from build123d import *

# Parameters (mm, degrees)
F0_W     = 8
F0_H     = 24
F1_DEPTH = 4
F2_DEPTH = 8
F3_W     = 16
F3_H     = 16
F4_DEPTH = 2


with BuildPart() as f1:
    # F0 (on Front) → F1 (new body, symmetric)
    with BuildSketch(Plane.XZ):
        with Locations((-4, 7)):
            Rectangle(F0_W, F0_H)
        with Locations((-12, 7)):
            Rectangle(F0_W, F0_H)
        with Locations((4, 7)):
            Rectangle(F0_W, F0_H)
        with Locations((12, 7)):
            Rectangle(F0_W, F0_H)
        with Locations((4, -17)):
            Rectangle(F0_W, F0_H)
        with Locations((-4, -17)):
            Rectangle(F0_W, F0_H)
    extrude(amount=F1_DEPTH, both=True)

    # F0 (on Front) → F2 (join, symmetric)
    with BuildSketch(Plane.XZ):
        Polygon((-8, 19), (0, 19), (8, 19), (8, 35), (-8, 35), align=None)
    extrude(amount=F2_DEPTH, both=True)

    # F3 (on face) → F4 (join)
    with BuildSketch(Plane(origin=(0, 0, -29), x_dir=(1, 0, 0), z_dir=(0, 0, -1))):
        Rectangle(F3_W, F3_H)
    extrude(amount=F4_DEPTH)


solid = f1.part
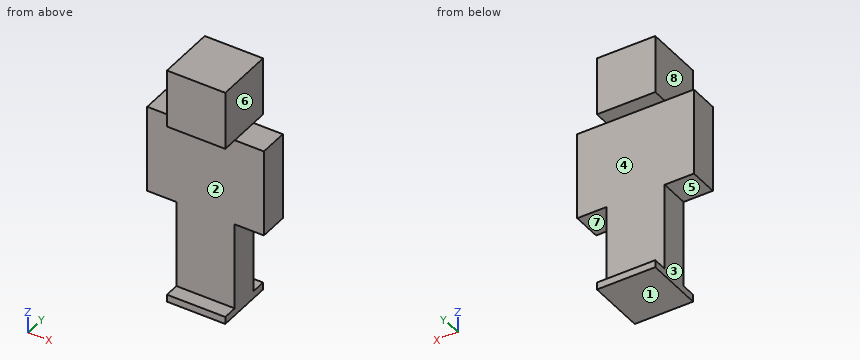
For this review, take the finished solid that the model builds, in its own axes (mm). Face numbers are marked on the shaded views. A direction names the side the tool comes from. Round coordinates to 2 decimals unless told otherwise and drop trailing zeros. Write each loop counter-clockwise with the first axis right and the second up, starting at its lowest first coordinate (ties: lowest second). Pieces come first, ordered by that corner, then holes. Notation, with made-up numbers: M 37.5,7.5 L 63.5,7.5 A31 ccw 63.5,46.5 Z; hole C -11,35.25 d3. An arc over 180 degrees is marked long. Write item = value, one per line. Start each with the question number.
(1) For the marked faces 4, 5, 6, 7 and 8, list the 3-axis set-ups (+Z, -Z, +X, -X, +Y, -Y) from which the entire face can be reached by the end or side of a thin tool; tool diameter is ignored.
(2) We need section B-B (x = 1.5). Give the boundary of the cut face in (y, z).
(3) Clearance check with flat-ended pins moving along their axes: pin 1 Ø16 at (x, z) = (-0.5, -8) entering from -Y; pin 2 Ø1.5 at (y, z) = (4.5, -15.5) entering from -X; pin 3 Ø4 at (x, y) = (10.5, 0) entering from -Z; pin 4 Ø6.5 at (x, y) = (10, 0.5) entering from +Z. State where each tip first meets the part, or that it passes through.
(4) We need section C-C (y = 2). Give the boundary of the cut face in (x, z), then the cut area to 3 significant figures.
(5) For line 1 along Z through (x, y) = (-6.5, -5.5); line 2 along Z through (x, y) = (10, 0.5); line 3 along X through (y, z) = (-3.75, 25), list the stretches that pass through material, from the lowest coordinate up.
(6) The part is to be moulded in two halves that separate along Z. For the marked faces 1, 2 and 3, say which applies: +Z half, -Z half, draft (parallel to the pull), parting line (faces both ways), or undercut.
(7) We need section A-A (y = 7). Give the boundary of the cut face in (x, z), then the cut area to 3 significant figures.
(8) We need section D-D (z = -8.5). Give the boundary of the cut face in (x, y), then the cut area to 3 significant figures.
Results found:
q1.face_4 = +X, -X, +Y
q1.face_5 = -Z, -X, +Y, -Y
q1.face_6 = +Z, +X, +Y, -Y
q1.face_7 = -Z, +X, +Y, -Y
q1.face_8 = +Z, -X, +Y, -Y
q2.outline = M -8,-31 L 8,-31 L 8,-29 L 4,-29 L 4,19 L 8,19 L 8,35 L -8,35 L -8,19 L -4,19 L -4,-29 L -8,-29 Z
q3.pin_1 = -4
q3.pin_2 = -8
q3.pin_3 = -5
q3.pin_4 = 35
q4.outline = M -16,-5 L -8,-5 L -8,-31 L 8,-31 L 8,-5 L 16,-5 L 16,19 L 8,19 L 8,35 L -8,35 L -8,19 L -16,19 Z
q4.area = 1,440 mm²
q5.line_1 = -31 to -29, 19 to 35
q5.line_2 = -5 to 19
q5.line_3 = -8 to 8
q6.face_1 = -Z half
q6.face_2 = undercut
q6.face_3 = draft
q7.outline = M -8,-31 L 8,-31 L 8,-29 L -8,-29 Z; M -8,19 L 8,19 L 8,35 L -8,35 Z
q7.area = 288 mm²
q8.outline = M -8,-4 L 8,-4 L 8,4 L -8,4 Z
q8.area = 128 mm²
